```python
from build123d import *

# Parameters (mm, degrees)
BASE_FLANGE1_DEPTH = 2.3
SKETCH6_W          = 3.35
SKETCH6_H          = 2.3
TAB1_DEPTH         = 2.3


# Sheet-metal steps are written as plain solids
with BuildPart() as part:
    # Model → Base-Flange1 (new body)
    with BuildSketch(Plane.XY):
        with BuildLine():
            Line((248.218742139, -402.267177227), (248.210301655, -402.327638653))
            Line((248.210301655, -402.327638653), (248.222510212, -402.491323752))
            add(Edge.make_bspline(
                [(248.222510212, -402.491323752), (248.246022989, -403.332056241), (248.70901563, -405.763218763), (249.319354503, -407.010912211)],
                knots=[15, 15, 15, 15, 16, 16, 16, 16], degree=3))
            add(Edge.make_bspline(
                [(249.319354503, -407.010912211), (249.523464167, -407.428166136), (250.554572065, -409.330398118), (251.019073512, -409.330398118)],
                knots=[16, 16, 16, 16, 17, 17, 17, 17], degree=3))
            Line((251.019073512, -409.330398118), (255.183497951, -409.330398118))
            add(Edge.make_bspline(
                [(255.183497951, -409.330398118), (255.57849992, -409.330398118), (256.903800339, -407.601307276), (257.216965505, -405.238012255)],
                knots=[18, 18, 18, 18, 19, 19, 19, 19], degree=3))
            add(Edge.make_bspline(
                [(257.216965505, -405.238012255), (257.282443851, -405.253687439), (257.400782881, -405.285511509), (257.476488854, -405.305880636)],
                knots=[19, 19, 19, 19, 20, 20, 20, 20], degree=3))
            add(Edge.make_bspline(
                [(257.476488854, -405.305880636), (258.053585412, -405.461039124), (259.01894423, -405.720627069), (260.177228396, -405.720627069)],
                knots=[20, 20, 20, 20, 21, 21, 21, 21], degree=3))
            add(Edge.make_bspline(
                [(260.177228396, -405.720627069), (261.701597021, -405.720627069), (263.091822241, -405.273152229), (264.309275921, -404.390604893)],
                knots=[21, 21, 21, 21, 22, 22, 22, 22], degree=3))
            add(Edge.make_bspline(
                [(264.309275921, -404.390604893), (266.463709447, -402.828426345), (266.962343955, -401.784562413), (267.352996251, -400.677050342)],
                knots=[22, 22, 22, 22, 23, 23, 23, 23], degree=3))
            add(Edge.make_bspline(
                [(267.352996251, -400.677050342), (267.416579794, -400.496828784), (267.462485692, -400.366647239), (267.523872987, -400.243872648)],
                knots=[23, 23, 23, 23, 24, 24, 24, 24], degree=3))
            add(Edge.make_bspline(
                [(267.523872987, -400.243872648), (267.937370572, -399.417178923), (270.638605347, -395.276389468), (271.926597358, -393.708698768)],
                knots=[24, 24, 24, 24, 25, 25, 25, 25], degree=3))
            add(Edge.make_bspline(
                [(271.926597358, -393.708698768), (273.376056688, -391.944379242), (276.34214037, -385.026811485), (275.876086264, -380.104114983)],
                knots=[25, 25, 25, 25, 26, 26, 26, 26], degree=3))
            add(Edge.make_bspline(
                [(275.876086264, -380.104114983), (275.8417645, -379.564656094), (274.799645491, -372.313924687), (269.70086935, -371.365600484)],
                knots=[0, 0, 0, 0, 1, 1, 1, 1], degree=3))
            add(Edge.make_bspline(
                [(269.70086935, -371.365600484), (269.207450344, -371.273829209), (264.137348452, -370.462620652), (260.904098088, -376.084398314)],
                knots=[1, 1, 1, 1, 2, 2, 2, 2], degree=3))
            add(Edge.make_bspline(
                [(260.904098088, -376.084398314), (260.433751909, -376.902207435), (257.516322771, -383.883501762), (257.032437578, -384.730177041)],
                knots=[2, 2, 2, 2, 3, 3, 3, 3], degree=3))
            add(Edge.make_bspline(
                [(257.032437578, -384.730177041), (256.627208222, -385.439479138), (256.175534672, -386.334514945), (255.738718096, -387.200052122)],
                knots=[3, 3, 3, 3, 4, 4, 4, 4], degree=3))
            add(Edge.make_bspline(
                [(255.738718096, -387.200052122), (255.500946273, -387.671364299), (255.11366392, -388.439088056), (254.863555112, -388.899096881)],
                knots=[4, 4, 4, 4, 5, 5, 5, 5], degree=3))
            add(Edge.make_bspline(
                [(254.863555112, -388.899096881), (254.791907734, -389.030873232), (254.698271896, -389.145280785), (254.58356807, -389.241931628)],
                knots=[5, 5, 5, 5, 6, 6, 6, 6], degree=3))
            add(Edge.make_bspline(
                [(254.58356807, -389.241931628), (254.060651196, -389.68254776), (253.251264748, -390.417536599), (252.487366168, -391.213071598)],
                knots=[6, 6, 6, 6, 7, 7, 7, 7], degree=3))
            add(Edge.make_bspline(
                [(252.487366168, -391.213071598), (250.221699122, -393.572574432), (249.853612202, -394.87055722), (249.773793646, -395.641655717)],
                knots=[7, 7, 7, 7, 8, 8, 8, 8], degree=3))
            add(Edge.make_bspline(
                [(249.773793646, -395.641655717), (249.748472194, -395.887075707), (249.70937036, -396.14291711), (249.667964619, -396.413744679)],
                knots=[8, 8, 8, 8, 9, 9, 9, 9], degree=3))
            add(Edge.make_bspline(
                [(249.667964619, -396.413744679), (249.5552028, -397.150487356), (249.42571589, -397.996549574), (249.530537872, -398.885487222)],
                knots=[9, 9, 9, 9, 10, 10, 10, 10], degree=3))
            add(Edge.make_bspline(
                [(249.530537872, -398.885487222), (249.565005835, -399.177791085), (249.489477062, -399.47455308), (249.322935943, -399.717233208)],
                knots=[10, 10, 10, 10, 11, 11, 11, 11], degree=3))
            add(Edge.make_bspline(
                [(249.322935943, -399.717233208), (248.372080781, -401.102798846), (248.260421691, -401.546272976), (248.227591728, -401.973655092)],
                knots=[11, 11, 11, 11, 12, 12, 12, 12], degree=3))
            add(Edge.make_bspline(
                [(248.227591728, -401.973655092), (248.223328422, -402.029207256), (248.218354566, -402.115851408), (248.218742139, -402.267177227)],
                knots=[12, 12, 12, 12, 13, 13, 13, 13], degree=3))
        make_face()
    extrude(amount=-BASE_FLANGE1_DEPTH)

    # Sketch6 → Tab1 (add)
    with BuildSketch(Plane.XY):
        with Locations((253.086490394, -410.480398118)):
            Rectangle(SKETCH6_W, SKETCH6_H)
    extrude(amount=-TAB1_DEPTH)


solid = part.part
```
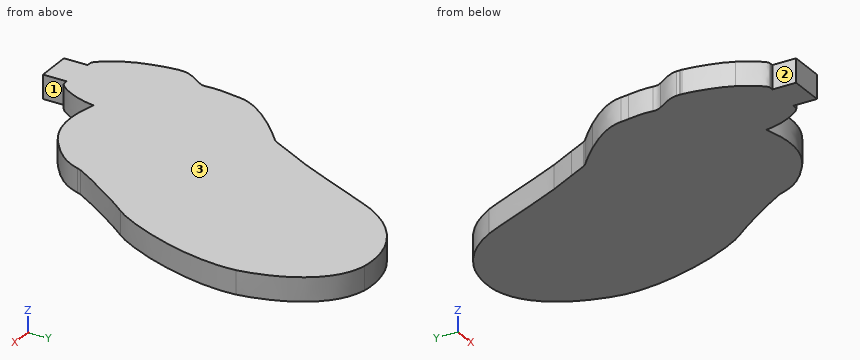
The listing builds one solid part. Answer for the finished solid, in the listing's coordinates (mm). Face numbers are marked on the shaded views. A direction names the side the tool comes from. Round coordinates to 2 decimals unless told otherwise and drop trailing zeros. Answer as CSV lines item,"result". Start each with the question number.
(1) A tool of negligible diameter and unlimited length cuts with its end or side. For the marked faces 1, 2 and 3, from which of +Z, -Z, +X, -X, +Y, -Y can it reach the whole face along a straight path? Write none if from no direction.
(2) Flat-ended cylindrical pins translate along their axes: pin 1 Ø3 at (x, y) = (252.5, -387.5) entering from -Z; pin 2 Ø1.1 at (y, z) = (-411, -1) entering from -X. Find the tip coordinate at first contact, or state that the pin passes through.
(3) Find the intervals of material crossed by probe 1 along Y at (x, z) = (260.5, -1.7); probe 2 along Y at (x, z) = (270.25, -0.4); probe 3 along X at (y, z) = (-395.5, -2), in increasing order. Write a range as from..to.
Evaluation:
1,face 1,"+Z, -Z, +X, -Y"
1,face 2,"+Z, -Z, -X, -Y"
1,face 3,"+Z, +X, -X, +Y, -Y"
2,pin 1,"through"
2,pin 2,"x = 251.41"
3,probe 1,"-405.71..-376.92"
3,probe 2,"-396..-371.5"
3,probe 3,"249.79..270.59"
